The listing builds one solid part. Answer for the finished solid, in the listing's coordinates (mm). A direction names the side the tool comes from. Give positions to 0.01 mm unless a question says otherwise; leave off trailing zeros. Order: outer loops, then holes, each group sorted by start corner. A loop starts at its lowest first (then second) coordinate and runs counter-clockwise, first axis right, second up. Notation, with made-up numbers: (88.5, 48) -> (136.5, 48) arc R9 ccw to (136.5, 60) -> close; hole circle Ø1 at (-17.5, 7.5). An arc over 180 degrees is marked (long way). Answer as a JSON object with one key per item and string values. Group by question number.
```python
from build123d import *

# Parameters (mm, degrees)
CROQUIS1_R              = 1.5
SALIENTE_EXTRUIR1_DEPTH = 3
CROQUIS2_W              = 20
CROQUIS2_H              = 3
SALIENTE_EXTRUIR2_DEPTH = 3


with BuildPart() as part:
    # Croquis1 → Saliente-Extruir1 (new body)
    with BuildSketch(Plane(origin=(0, 0, 0), x_dir=(1, 0, 0), z_dir=(0, 1, 0))):
        with BuildLine():
            Line((20, -10), (-20, -10))
            ThreePointArc((-20, -10), (-23.535533906, -8.535533906), (-25, -5))
            Line((-25, -5), (-25, 10))
            Line((-25, 10), (25, 10))
            Line((25, 10), (25, -5))
            ThreePointArc((25, -5), (23.535533906, -8.535533906), (20, -10))
        make_face()
        with Locations(Location((0, 0, 0), (0, 0, 270))):
            Circle(CROQUIS1_R, mode=Mode.SUBTRACT)
    extrude(amount=SALIENTE_EXTRUIR1_DEPTH)

    # Croquis2 → Saliente-Extruir2 (add)
    with BuildSketch(Plane(origin=(0, 0, -10), x_dir=(-1, 0, 0), z_dir=(0, 0, -1))):
        with Locations((0, 1.5)):
            Rectangle(CROQUIS2_W, CROQUIS2_H)
    extrude(amount=SALIENTE_EXTRUIR2_DEPTH)


solid = part.part
```
(1) Find the intervals of material crossed by line 1 along X through (y, z) = (1.8, 0); line 2 along Z through (x, y) = (16.5, 1.7); line 3 along X through (y, z) = (1.4, -0.5), in increasing order. Write a range as [from, to].
(2) A flat-ended cylindrical pin translates along its axis: pin 1 Ø1.5 at (x, y) = (-21, 1) entering from -Z. Find the tip coordinate at first contact, or state that the pin passes through.
(3) A cutting plane is placed at A-A (y = 1.1). Determine the outline of the cut face in (x, z).
(4) A cutting plane is placed at C-C (z = 0). Determine the outline of the cut face in (x, y), and give its area (3 significant figures).
(5) Which of the six approach directions +Z, -Z, +X, -X, +Y, -Y give full straight-line access (tool end or side, diameter ignored) to faces 1 (the flat face through (-10, 1, -11)), 2 (the flat face through (0, 3, -2)), 3 (the flat face through (10, 1, -11))?
(6) A cutting plane is placed at B-B (x = 0). Determine the outline of the cut face in (y, z), and give its area (3 significant figures).
(7) For a pull along X with two mould halves and no side action, classify faces 4 (the flat face through (-25, 1, -2)), 5 (the cylindrical face through (0.45, 1.48, 1.43)), 6 (the flat face through (25, 1, -3)), 7 (the flat face through (-18, 1, -10)) as +X half, -X half, draft (parallel to the pull), parting line (faces both ways), or undercut.
(8) A cutting plane is placed at D-D (x = 18). Determine the outline of the cut face in (y, z), and give its area (3 significant figures).
Check sheet entries:
{
 "1": {"line 1": "x = [-25, -1.5], [1.5, 25]", "line 2": "z = [-10, 10]", "line 3": "x = [-25, -1.41], [1.41, 25]"},
 "2": {"pin 1": "stops at z = -10"},
 "3": {"outline": "(-25, -10) -> (-10, -10) -> (-10, -13) -> (10, -13) -> (10, -10) -> (25, -10) -> (25, 5) arc R5 ccw to (20, 10) -> (-20, 10) arc R5 ccw to (-25, 5) -> close; hole circle Ø3 at (0, 0)"},
 "4": {"outline": "(-25, 0) -> (-1.5, 0) -> (-1.5, 3) -> (-25, 3) -> close; (1.5, 0) -> (25, 0) -> (25, 3) -> (1.5, 3) -> close", "area": "141 mm2"},
 "5": {"face 1": "-Z, -X, +Y, -Y", "face 2": "+Z, -Z, +X, -X, +Y", "face 3": "-Z, +X, +Y, -Y"},
 "6": {"outline": "(0, -13) -> (3, -13) -> (3, -1.5) -> (0, -1.5) -> close; (0, 1.5) -> (3, 1.5) -> (3, 10) -> (0, 10) -> close", "area": "60.0 mm2"},
 "7": {"face 4": "-X half", "face 5": "undercut", "face 6": "+X half", "face 7": "draft"},
 "8": {"outline": "(0, -10) -> (3, -10) -> (3, 10) -> (0, 10) -> close", "area": "60.0 mm2"}
}
